```python
from build123d import *

# Parameters (mm, degrees)
SKETCH1_R           = 28.1
BOSS_EXTRUDE2_DEPTH = 61.3
SKETCH3_R           = 18.6
CUT_EXTRUDE2_DEPTH  = 58.8
SKETCH4_W           = 56.2
SKETCH4_H           = 56.2
BOSS_EXTRUDE3_DEPTH = 56.2
SKETCH5_R           = 16.1
CUT_EXTRUDE4_DEPTH  = 5
SKETCH6_W           = 49.797391422
SKETCH6_H           = 49.779255452
CUT_EXTRUDE5_DEPTH  = 53.7
SKETCH7_R           = 28.1
BOSS_EXTRUDE4_DEPTH = 321.5
CUT_EXTRUDE6_DEPTH  = 10
SKETCH9_R           = 3
CUT_EXTRUDE7_DEPTH  = 1
SKETCH10_R          = 6.025
CUT_EXTRUDE8_DEPTH  = 0.1
SKETCH18_R          = 3.75
CUT_EXTRUDE9_DEPTH  = 100
SKETCH19_R          = 3.75
CUT_EXTRUDE11_DEPTH = 325
SKETCH20_W          = 86.001348001
SKETCH20_H          = 379.283348588
CUT_EXTRUDE16_DEPTH = 171.5


with BuildPart() as part:
    # Sketch1 → Boss-Extrude2 (new body)
    with BuildSketch(Plane.XY):
        Circle(SKETCH1_R)
    extrude(amount=BOSS_EXTRUDE2_DEPTH)

    # Sketch3 → Cut-Extrude2 (cut)
    with BuildSketch(Plane.XY.offset(61.3)):
        with Locations((0, -7)):
            Circle(SKETCH3_R)
    extrude(amount=-CUT_EXTRUDE2_DEPTH, mode=Mode.SUBTRACT)

    # Sketch4 → Boss-Extrude3 (add)
    with BuildSketch(Plane(origin=(0, 0, 0), x_dir=(-1, 0, 0), z_dir=(0, 0, -1))):
        Rectangle(SKETCH4_W, SKETCH4_H)
    extrude(amount=BOSS_EXTRUDE3_DEPTH)

    # Sketch5 → Cut-Extrude4 (cut)
    with BuildSketch(Plane.XY.offset(2.5)):
        with Locations((0, -7)):
            Circle(SKETCH5_R)
    extrude(amount=-CUT_EXTRUDE4_DEPTH, mode=Mode.SUBTRACT)

    # Sketch6 → Cut-Extrude5 (cut)
    with BuildSketch(Plane(origin=(0, 0, -56.2), x_dir=(-1, 0, 0), z_dir=(0, 0, -1))):
        Rectangle(SKETCH6_W, SKETCH6_H)
    extrude(amount=-CUT_EXTRUDE5_DEPTH, mode=Mode.SUBTRACT)

    # Sketch7 → Boss-Extrude4 (add)
    with BuildSketch(Plane(origin=(0, -28.1, 0), x_dir=(-1, 0, 0), z_dir=(0, -1, 0))):
        with Locations(Location((0, 28.1, 0), (0, 0, 90))):
            Circle(SKETCH7_R)
    extrude(amount=BOSS_EXTRUDE4_DEPTH)

    # Sketch8 → Cut-Extrude6 (cut)
    with BuildSketch(Plane(origin=(0, -349.6, 0), x_dir=(-1, 0, 0), z_dir=(0, -1, 0))):
        with BuildLine():
            Line((-1.658312395, 25.832078896), (1.658312395, 25.832078896))
            ThreePointArc((1.658312395, 25.832078896), (3, 28.332078896), (1.658312395, 30.832078896))
            Line((1.658312395, 30.832078896), (-1.658312395, 30.832078896))
            ThreePointArc((-1.658312395, 30.832078896), (-3, 28.332078896), (-1.658312395, 25.832078896))
        make_face()
    extrude(amount=-CUT_EXTRUDE6_DEPTH, mode=Mode.SUBTRACT)

    # Sketch9 → Cut-Extrude7 (cut)
    with BuildSketch(Plane(origin=(0, -349.6, 0), x_dir=(-1, 0, 0), z_dir=(0, -1, 0))):
        with Locations(Location((0, 28.332078896, 0), (0, 0, 90))):
            Circle(SKETCH9_R)
    extrude(amount=-CUT_EXTRUDE7_DEPTH, mode=Mode.SUBTRACT)

    # Sketch10 → Cut-Extrude8 (cut)
    with BuildSketch(Plane(origin=(0, -349.6, 0), x_dir=(-1, 0, 0), z_dir=(0, -1, 0))):
        with Locations(Location((0, 28.332078896, 0), (0, 0, 90))):
            Circle(SKETCH10_R)
    extrude(amount=-CUT_EXTRUDE8_DEPTH, mode=Mode.SUBTRACT)

    # Cut-Sweep4: sweep along a path in Sketch15
    with BuildLine(Plane(origin=(0, -349.6, 0), x_dir=(-1, 0, 0), z_dir=(0, -1, 0))) as cut_sweep4_path:
        ThreePointArc((15, 28.332078896), (0, 43.332078896), (-15, 28.332078896))
    # 3DSketch2 → Cut-Sweep4 (sweep, cut)
    with BuildSketch(Plane(origin=(-15, -349.6, -28.332078896), x_dir=(-0.022748965612757834, 0.999741208795331, 0), z_dir=(0, 0, 1))):
        Polygon((0, 0), (0.170617242, 7.498059066), (329.685319661, 0), (329.514702419, -7.498059066), align=None)
    sweep(path=cut_sweep4_path.line, mode=Mode.SUBTRACT)

    # Sketch18 → Cut-Extrude9 (cut)
    with BuildSketch(Plane.XY.offset(61.3)):
        with Locations((0, 18.75)):
            Circle(SKETCH18_R)
    extrude(amount=-CUT_EXTRUDE9_DEPTH, mode=Mode.SUBTRACT)

    # Sketch19 → Cut-Extrude11 (cut)
    with BuildSketch(Plane(origin=(0, -349.6, 0), x_dir=(-1, 0, 0), z_dir=(0, -1, 0))):
        with Locations((-18.75, 28.332078896)):
            Circle(SKETCH19_R)
        with Locations((18.75, 28.332078896)):
            Circle(SKETCH19_R)
    extrude(amount=-CUT_EXTRUDE11_DEPTH, mode=Mode.SUBTRACT)

    # Sketch20 → Cut-Extrude16 (cut)
    with BuildSketch(Plane(origin=(0, 0, -56.2), x_dir=(-1, 0, 0), z_dir=(0, 0, -1))):
        with Locations((14.900674001, -217.741674294)):
            Rectangle(SKETCH20_W, SKETCH20_H)
    extrude(amount=-CUT_EXTRUDE16_DEPTH, mode=Mode.SUBTRACT)


solid = part.part
```
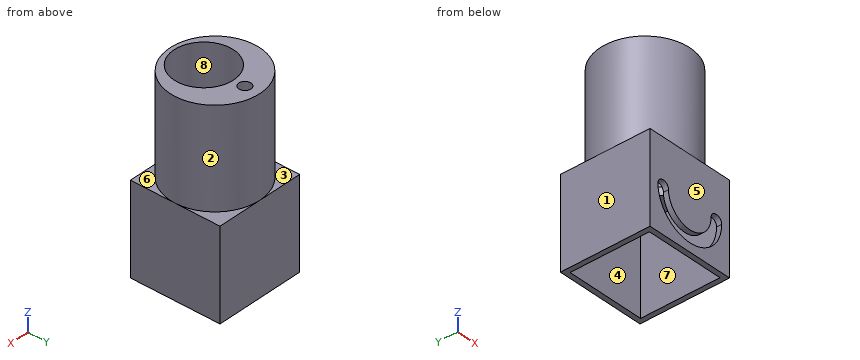
Input: part model. Units: mm. Frame: model coordinates. Face numbers are marked on the shaded views. A direction names the side the tool comes from. Round coordinates to 2 decimals unless told otherwise and drop trailing zeros. Loops run counter-clockwise (first coordinate to the right, second up) from the corner with the lowest first, then second, coordinate; pieces in that order, holes last. Notation, with made-up numbers: (45.5, 19.25) -> (50.5, 19.25) arc R21 cw to (50.5, 30.25) -> close; hole circle Ø6 at (5.25, 46). An arc over 180 degrees is marked (long way). Use one line per item in the form item = value. Start each with the question number.
Item 1: Material intervals for L1, parallel to Y at x = 0, z = 45.5; L2, parallel to Y at x = 0, z = -1.4; L3, parallel to X at y = 24.5, z = -39.5, sorted ascending. Write a range as from..to.
Item 2: Contact query for flat-ended pins moving along their axis: pin 1 Ø2 at (x, z) = (19.5, 19.5) entering from -Y; pin 2 Ø10 at (y, z) = (-9, 35.5) entering from +X; pin 3 Ø10 at (x, y) = (0, 18.75) entering from -Z. Output: stop coordinate, or through.
Item 3: Section query A-A on y = -18. Return the cut outline in (x, z), then the cut area to 3 significant figures.
Item 4: Section query C-C on x = -2. Return the cut outline in (y, z), then the cut area to 3 significant figures.
Item 5: Mould query, pull axis Y, two halves, no side actions, for the marked faces 5, 6, 7 and 8. Classes: pulls with the +Y half, pulls with the -Y half, needs draft (parallel to the pull), parting line crosses it, or undercut.
Item 6: Section query D-D on z = 24. Return the cut outline in (x, y).
Item 7: Set-up query: the marked faces 1, 2, 3 and 4. Return all of +Z, -Z, +X, -X, +Y, -Y with unobstructed straight access to the full face (end or side cutting, diameter ignored); none if empty.
Item 8: Section query B-B on z = -14. Return the cut outline in (x, y), then the cut area to 3 significant figures.
Ans:
q1.L1 = -28.1..-25.6, 11.6..15, 22.5..28.1
q1.L2 = -28.1..-23.1, 9.1..15, 22.5..28.1
q1.L3 = -28.1..-24.9, 24.9..28.1
q2.pin_1 = -21.15
q2.pin_2 = 27.81
q2.pin_3 = -2.5
q3.outline = (-28.1, -56.2) -> (-24.9, -56.2) -> (-24.9, -2.5) -> (-11.76, -2.5) -> (-11.76, 2.5) -> (-15, 2.5) -> (-15, 61.3) -> (-21.58, 61.3) -> (-21.58, 0) -> (-28.1, 0) -> close; (11.76, -2.5) -> (24.9, -2.5) -> (24.9, -56.2) -> (28.1, -56.2) -> (28.1, 0) -> (21.58, 0) -> (21.58, 61.3) -> (15, 61.3) -> (15, 2.5) -> (11.76, 2.5) -> close
q3.area = 1,250 mm^2
q4.outline = (-28.1, -56.2) -> (-24.89, -56.2) -> (-24.89, -50.74) -> (-28.1, -50.74) -> close; (-28.1, -43.2) -> (-24.89, -43.2) -> (-24.89, -2.5) -> (-22.98, -2.5) -> (-22.98, 2.5) -> (-25.49, 2.5) -> (-25.49, 61.3) -> (-28.03, 61.3) -> (-28.03, 0) -> (-28.1, 0) -> close; (8.98, -2.5) -> (15.58, -2.5) -> (15.58, 61.3) -> (11.49, 61.3) -> (11.49, 2.5) -> (8.98, 2.5) -> close; (21.92, -2.5) -> (24.89, -2.5) -> (24.89, -56.2) -> (28.1, -56.2) -> (28.1, 0) -> (28.03, 0) -> (28.03, 61.3) -> (21.92, 61.3) -> close
q4.area = 1,160 mm^2
q5.face_5 = pulls with the -Y half
q5.face_6 = needs draft
q5.face_7 = undercut
q5.face_8 = undercut
q6.outline = circle Ø56.2 at (0, 0); hole circle Ø37.2 at (0, -7); hole circle Ø7.5 at (0, 18.75)
q7.face_1 = +Z, -Z, -X, +Y, -Y
q7.face_2 = +Z
q7.face_3 = +Z, -X, +Y
q7.face_4 = -Z
q8.outline = (-28.1, -28.1) -> (28.1, -28.1) -> (28.1, 28.1) -> (-28.1, 28.1) -> close; hole (-24.9, -24.89) -> (24.9, -24.89) -> (24.9, 24.89) -> (-24.9, 24.89) -> close
q8.area = 680 mm^2
